For this review, take the finished solid that the model builds, in its own axes (mm). Face numbers are marked on the shaded views. A direction names the side the tool comes from. Coordinates: 2 decimals unless noted, no trailing zeros. Order: outer loops, then holes, each group sorted by start corner. A loop starts at its lowest first (then second) coordinate and runs counter-clockwise, first axis right, second up. Notation, with made-up numbers: (-23, 57) -> (-18, 57) arc R28 ccw to (-18, 94) -> close; hole circle Ø8 at (73.5, 10.5). An arc over 180 degrees is marked (long way). Write item = value, one per line. Start each with the question number.
1) Wall thickness on probe 1 along X at (y, z) = (108, 0); probe 2 along X at (y, z) = (29.5, 2); probe 3 along Z at (x, y) = (-2, 120.5): over which ranges is each line inside the solid? List them lowest first. Write a range as [from, to].
2) Consider section D-D on z = -56. Give the boundary of the cut face in (x, y).
3) Draft analysis for pull direction X (two halves, no side actions). For the marked faces 3, 4 and 5, state which applies: +X half, -X half, draft (parallel to the pull), parting line (faces both ways), or undercut.
4) Consider section A-A on z = 0. Give the boundary of the cut face in (x, y), and give its area (3 significant figures).
5) Consider section B-B on x = 0. Give the boundary of the cut face in (y, z).
6) Machinability: for the marked faces 1 and 2, which of the approach directions +Z, -Z, +X, -X, +Y, -Y give a long, thin tool a straight path to every point of the face, cutting with its end or side? Answer none if there is none.
7) Consider section C-C on y = 39. Give the boundary of the cut face in (x, z), and give its area (3 significant figures).
8) Insertion check: pin 1 Ø6 at (y, z) = (66.5, -29) entering from -X; pin 2 Ø1.5 at (y, z) = (112, -44.5) entering from +X; pin 3 Ø8 at (y, z) = (78, -54.5) entering from -X; pin 4 Ø3 at (y, z) = (101.5, 3) entering from -X. Each pin has a flat end and moves straight along its axis. Give the tip position at first contact, or say it passes through.
from build123d import *

# Parameters (mm, degrees)
BOSS_EXTRUDE1_DEPTH = 100
SKETCH3_R           = 50
BOSS_EXTRUDE3_DEPTH = 80
CHAMFER1_SIZE       = 5
FILLET1_R           = 1
SKETCH4_R           = 5
CUT_EXTRUDE1_DEPTH  = 20
SKETCH5_R           = 15
SKETCH5_R_2         = 2.5
SKETCH5_W           = 60
SKETCH5_H           = 10
SKETCH5_W_2         = 50
CUT_EXTRUDE2_DEPTH  = 20
SKETCH6_W           = 150
SKETCH6_H           = 200
CUT_EXTRUDE3_DEPTH  = 181
SKETCH7_R           = 83.3335
BOSS_EXTRUDE4_DEPTH = 30
SHELL1_T            = -4
SKETCH10_R          = 5
CUT_EXTRUDE4_DEPTH  = 209


with BuildPart() as part:
    # Sketch2 → Boss-Extrude1 (new, symmetric)
    with BuildSketch(Plane.XY):
        with BuildLine():
            Line((-75, 50), (-70, 50))
            ThreePointArc((-70, 50), (-65, 45), (-60, 50))
            Line((-60, 50), (-35, 50))
            Line((-35, 50), (-25, 50))
            Line((-25, 50), (25, 50))
            Line((25, 50), (35, 50))
            Line((35, 50), (60, 50))
            ThreePointArc((60, 50), (65, 45), (70, 50))
            Line((70, 50), (75, 50))
            Line((75, 50), (75, 15))
            ThreePointArc((75, 15), (70.980762114, 0), (75, -15))
            Line((75, -15), (75, -50))
            Line((75, -50), (70, -50))
            ThreePointArc((70, -50), (65, -45), (60, -50))
            Line((60, -50), (35, -50))
            ThreePointArc((35, -50), (30, -45), (25, -50))
            Line((25, -50), (-25, -50))
            ThreePointArc((-25, -50), (-30, -45), (-35, -50))
            Line((-35, -50), (-60, -50))
            ThreePointArc((-60, -50), (-65, -45), (-70, -50))
            Line((-70, -50), (-75, -50))
            Line((-75, -50), (-75, -15))
            ThreePointArc((-75, -15), (-70.980762114, 0), (-75, 15))
            Line((-75, 15), (-75, 50))
        make_face()
    extrude(amount=BOSS_EXTRUDE1_DEPTH, both=True)

    # Sketch3 → Boss-Extrude3 (add)
    with BuildSketch(Plane(origin=(0, 50, 0), x_dir=(1, 0, 0), z_dir=(0, 1, 0))):
        with Locations(Location((0, 0, 0), (0, 0, 90))):
            Circle(SKETCH3_R)
    extrude(amount=BOSS_EXTRUDE3_DEPTH)

    # Chamfer1
    chamfer1_edges = [part.edges().sort_by_distance(p)[0] for p in [
        (0, 130, 50),
    ]]
    chamfer(chamfer1_edges, length=CHAMFER1_SIZE)

    # Fillet1
    fillet1_edges = [part.edges().sort_by_distance(p)[0] for p in [
        (-75, -50, 0),
        (-75, 50, 0),
        (75, 50, 0),
        (75, -50, 0),
    ]]
    fillet(fillet1_edges, radius=FILLET1_R)

    # Sketch4 → Cut-Extrude1 (cut)
    with BuildSketch(Plane.XZ.offset(50)):
        with Locations(Location((-47.5, 80, 0), (0, 0, 270))):
            Circle(SKETCH4_R)
        with Locations(Location((47.5, 80, 0), (0, 0, 270))):
            Circle(SKETCH4_R)
        with Locations(Location((47.5, 40, 0), (0, 0, 270))):
            Circle(SKETCH4_R)
        with Locations(Location((47.5, 0, 0), (0, 0, 270))):
            Circle(SKETCH4_R)
        with Locations(Location((47.5, -40, 0), (0, 0, 270))):
            Circle(SKETCH4_R)
        with Locations(Location((47.5, -80, 0), (0, 0, 270))):
            Circle(SKETCH4_R)
        with Locations(Location((-47.5, 40, 0), (0, 0, 270))):
            Circle(SKETCH4_R)
        with Locations(Location((-47.5, 0, 0), (0, 0, 270))):
            Circle(SKETCH4_R)
        with Locations(Location((-47.5, -40, 0), (0, 0, 270))):
            Circle(SKETCH4_R)
        with Locations(Location((-47.5, -80, 0), (0, 0, 270))):
            Circle(SKETCH4_R)
    extrude(amount=-CUT_EXTRUDE1_DEPTH, mode=Mode.SUBTRACT)

    # Sketch5 → Cut-Extrude2 (cut)
    with BuildSketch(Plane(origin=(0, 0, -100), x_dir=(-1, 0, 0), z_dir=(0, 0, -1))):
        with Locations((40, 25)):
            Circle(SKETCH5_R)
        with Locations((35, 25)):
            Circle(SKETCH5_R_2, mode=Mode.SUBTRACT)
        with Locations((45, 25)):
            Circle(SKETCH5_R_2, mode=Mode.SUBTRACT)
        with Locations((-25, -20)):
            Rectangle(SKETCH5_W, SKETCH5_H)
        with Locations((-25, 10)):
            Rectangle(SKETCH5_W_2, SKETCH5_H)
    extrude(amount=-CUT_EXTRUDE2_DEPTH, mode=Mode.SUBTRACT)

    # Sketch6 → Cut-Extrude3 (cut)
    with BuildSketch(Plane(origin=(0, 50, 0), x_dir=(1, 0, 0), z_dir=(0, 1, 0))):
        Rectangle(SKETCH6_W, SKETCH6_H)
    extrude(amount=-CUT_EXTRUDE3_DEPTH, mode=Mode.SUBTRACT)

    # Sketch7 → Boss-Extrude4 (add)
    with BuildSketch(Plane.XZ.offset(-50)):
        with Locations(Location((0, 0, 0), (0, 0, 270))):
            Circle(SKETCH7_R)
    extrude(amount=BOSS_EXTRUDE4_DEPTH)

    # Shell1
    shell1_openings = [part.faces().sort_by_distance(p)[0] for p in [
        (0, 20, 0),
    ]]
    offset(amount=SHELL1_T, openings=shell1_openings, kind=Kind.INTERSECTION)

    # Sketch10 → Cut-Extrude4 (cut)
    with BuildSketch(Plane(origin=(0, 130, 0), x_dir=(1, 0, 0), z_dir=(0, 1, 0))):
        with Locations(Location((0, 0, 0), (0, 0, 270))):
            Circle(SKETCH10_R)
    extrude(amount=-CUT_EXTRUDE4_DEPTH, mode=Mode.SUBTRACT)


solid = part.part
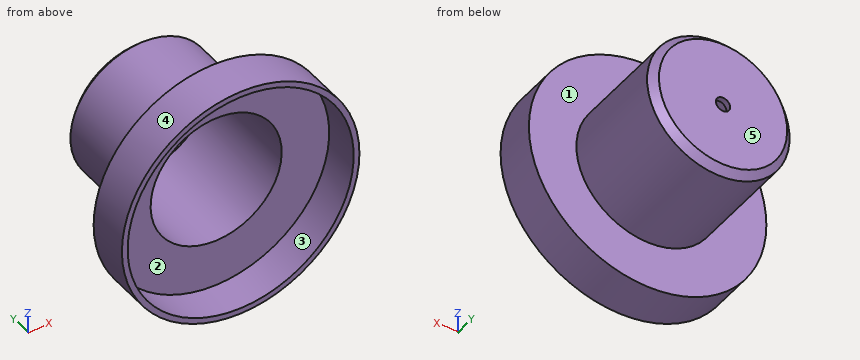
Answer sheet:
q1.probe_1 = [-50, -46], [46, 50]
q1.probe_2 = [-83.31, -79.31], [79.31, 83.31]
q1.probe_3 = [-49.96, -45.96], [45.96, 49.96]
q2.outline = (-61.71, 20) -> (-56.19, 20) -> (-56.19, 46) -> (56.19, 46) -> (56.19, 20) -> (61.71, 20) -> (61.71, 50) -> (-61.71, 50) -> close
q3.face_3 = undercut
q3.face_4 = parting line
q3.face_5 = draft
q4.outline = (-83.33, 20) -> (-79.33, 20) -> (-79.33, 46) -> (-46, 46) -> (-46, 123.34) -> (-43.34, 126) -> (-5, 126) -> (-5, 130) -> (-45, 130) -> (-50, 125) -> (-50, 50) -> (-83.33, 50) -> close; (5, 126) -> (43.34, 126) -> (46, 123.34) -> (46, 46) -> (79.33, 46) -> (79.33, 20) -> (83.33, 20) -> (83.33, 50) -> (50, 50) -> (50, 125) -> (45, 130) -> (5, 130) -> close
q4.area = 1,460 mm2
q5.outline = (20, -83.33) -> (50, -83.33) -> (50, -50) -> (125, -50) -> (130, -45) -> (130, -5) -> (126, -5) -> (126, -43.34) -> (123.34, -46) -> (46, -46) -> (46, -79.33) -> (20, -79.33) -> close; (20, 79.33) -> (46, 79.33) -> (46, 46) -> (123.34, 46) -> (126, 43.34) -> (126, 5) -> (130, 5) -> (130, 45) -> (125, 50) -> (50, 50) -> (50, 83.33) -> (20, 83.33) -> close
q6.face_1 = +Y
q6.face_2 = -Y
q7.outline = circle Ø166.67 at (0, 0); hole circle Ø158.67 at (0, 0)
q7.area = 2,040 mm2
q8.pin_1 = -42.71
q8.pin_2 = 24.21
q8.pin_3 = through
q8.pin_4 = -49.98
